Check sheet for the modelled part. Datum: model origin and axes. Units: mm. Coordinates: 2 decimals unless noted, no trailing zeros. Loops run counter-clockwise (first coordinate to the right, second up) from the corner with the lowest first, then second, coordinate; pieces in that order, holes last. Notation, with made-up numbers: M 85,74 L 95,74 A15 ccw 95,100 Z; hole C 8.25,58.25 d4. An arc over 180 degrees is marked long. Return JSON: item names as keys, results as strings.
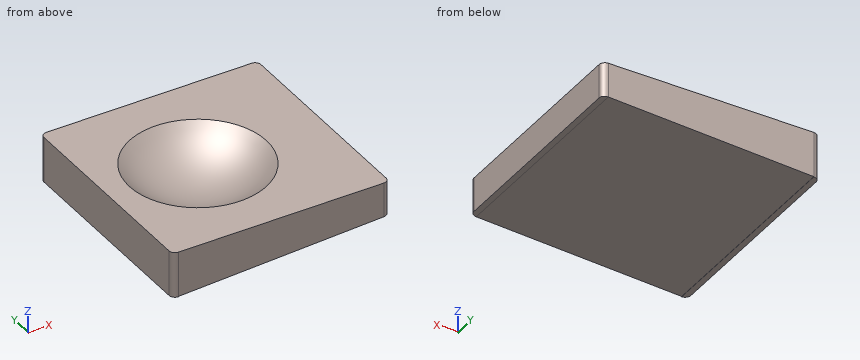
from build123d import *

# Parameters (mm, degrees)
F1_DEPTH = 4
F3_DEPTH = 19


with BuildPart() as f1:
    # F0 (on Top) → F1 (new body)
    with BuildSketch(Plane.XY):
        with BuildLine():
            ThreePointArc((9.5, 9), (9.3535533906, 9.3535533906), (9, 9.5))
            Line((9, 9.5), (-9, 9.5))
            ThreePointArc((-9, 9.5), (-9.3535533906, 9.3535533906), (-9.5, 9))
            Line((-9.5, 9), (-9.5, -9))
            ThreePointArc((-9.5, -9), (-9.3535533906, -9.3535533906), (-9, -9.5))
            Line((-9, -9.5), (9, -9.5))
            ThreePointArc((9, -9.5), (9.3535533906, -9.3535533906), (9.5, -9))
            Line((9.5, -9), (9.5, 9))
        make_face()
    extrude(amount=F1_DEPTH)

    # F2 (on face) → F3 (cut, through all)
    with BuildSketch(Plane.XZ.offset(9.5)):
        Polygon((9, 0.9736842105), (-9, 0.0263157895), (-9, 0), (9, 0), align=None)
        Polygon((9.5, 1), (9, 0.9736842105), (9, 0), (9.5, 0), align=None)
    extrude(amount=-F3_DEPTH, mode=Mode.SUBTRACT)

    # F4 (on Front) → F5 (revolve, cut)
    with BuildSketch(Plane.XZ):
        with BuildLine():
            Line((-1.5, 4), (-7.5, 4))
            ThreePointArc((-7.5, 4), (-4.75, 2.15), (-1.5, 1.5))
            Line((-1.5, 1.5), (-1.5, 4))
        make_face()
    revolve(axis=Axis((-1.5, 0, 2.3585720337), (0, 0, -1)), mode=Mode.SUBTRACT)


solid = f1.part
1) Go/stop test with a flat-tipped pin: pin 1 Ø3 at (x, y) = (-1.5, 7.5) entering from -Z. Record where the tip stops, or that it passes through.
Answers:
{"pin 1": "z = 0.34"}
2) Section check D-D on z = 0.6. Record the cut outline in (x, y), then the cut area to 3 significant figures.
Answers:
{"outline": "M -9.5,-9 A0.5 ccw -9,-9.5 L 1.9,-9.5 L 1.9,9.5 L -9,9.5 A0.5 ccw -9.5,9 Z", "area": "216 mm²"}
3) Scan lines: line 1 along X through (y, z) = (4.25, 3.2); line 2 along X through (y, z) = (-1, 2.4); line 3 along Y through (x, z) = (2, 3.1). Record each from-to range of solid material in increasing order. Write a range as [from, to].
Answers:
{"line 1": "[-9.5, -4.29], [1.29, 9.5]", "line 2": "[-9.5, -5.16], [2.16, 9.5]", "line 3": "[-9.5, -3.5], [3.5, 9.5]"}
4) Section check C-C on x = 0.25. Record the cut outline in (y, z).
Answers:
{"outline": "M -9.5,0.51 L 9.5,0.51 L 9.5,4 L 5.74,4 A8.27 cw -5.74,4 L -9.5,4 Z"}
5) Section check B-B on z = 1.75. Record the cut outline in (x, y).
Answers:
{"outline": "M -9.5,-9 A0.5 ccw -9,-9.5 L 9,-9.5 A0.5 ccw 9.5,-9 L 9.5,9 A0.5 ccw 9,9.5 L -9,9.5 A0.5 ccw -9.5,9 Z; hole C -1.5,0 d4.08"}
